```python
from build123d import *

# Parameters (mm, degrees)
F1_DEPTH = 10
F2_SIZE  = 5
F3_R     = 2.5
F4_DEPTH = 10
F5_R     = 1.5
F6_DEPTH = 12


with BuildPart() as f1:
    # F0 (on Front) → F1 (new body)
    with BuildSketch(Plane.XZ):
        with BuildLine():
            Line((-7, 0), (0, 0))
            Line((0, 0), (0, 30))
            Line((0, 30), (-20, 30))
            Line((-20, 30), (-20, 0))
            Line((-20, 0), (-13, 0))
            Line((-13, 0), (-13, 19.427699))
            ThreePointArc((-13, 19.427699), (-9.474739, 21.19446), (-7, 18.124513))
            Line((-7, 18.124513), (-7, 0))
        make_face()
    extrude(amount=F1_DEPTH)

    # F2
    f2_edges = [f1.edges().sort_by_distance(p)[0] for p in [
        (0, -5, 30),
        (-20, -5, 30),
    ]]
    chamfer(f2_edges, length=F2_SIZE)

    # F3 (on face) → F4 (cut)
    with BuildSketch(Plane.YZ):
        with Locations((-5, 16.878698)):
            Circle(F3_R)
        with Locations((-5, 7.148258)):
            Circle(F3_R)
    extrude(amount=-F4_DEPTH, mode=Mode.SUBTRACT)

    # F5 (on Front) → F6 (cut)
    with BuildSketch(Plane.XZ):
        with Locations((-16.984137, 21.757886)):
            Circle(F5_R)
        with Locations((-16.821511, 6.757886)):
            Circle(F5_R)
    extrude(amount=F6_DEPTH, mode=Mode.SUBTRACT)


solid = f1.part
```
Check sheet for the modelled part. Datum: model origin and axes. Units: mm. A direction names the side the tool comes from. Round coordinates to 2 decimals unless told otherwise and drop trailing zeros. Order: outer loops, then holes, each group sorted by start corner. A loop starts at its lowest first (then second) coordinate and runs counter-clockwise, first axis right, second up. Notation, with made-up numbers: (61, 58) - (101, 58) arc R24 cw to (101, 81) - close; hole circle Ø2 at (15, -31.75). An arc over 180 degrees is marked (long way). Write item = value, one per line.
Q1. Thickness scan on line 1 along Z through (x, y) = (-4.25, -5); line 2 along Z through (x, y) = (-4, -5); line 3 along X through (y, z) = (-4, 10.75). Record the ranges inside material, lowest first.
Computed:
line_1 = 0 to 4.65, 9.65 to 14.38, 19.38 to 29.25
line_2 = 0 to 4.65, 9.65 to 14.38, 19.38 to 29
line_3 = -20 to -13, -7 to 0
Q2. Section check C-C (x = -17.25). Record the boundary of the cut face in (y, z).
Computed:
outline = (-10, 0) - (0, 0) - (0, 5.32) - (-10, 5.32) - close; (-10, 8.2) - (0, 8.2) - (0, 20.28) - (-10, 20.28) - close; (-10, 23.23) - (0, 23.23) - (0, 27.75) - (-10, 27.75) - close
Q3. Section check B-B (y = -5). Record the boundary of the cut face in (x, z), and give its area (3 significant figures).
Computed:
outline = (-20, 0) - (-13, 0) - (-13, 19.43) arc R3.14 cw to (-7.26, 19.38) - (0, 19.38) - (0, 25) - (-5, 30) - (-15, 30) - (-20, 25) - close; (-7, 0) - (0, 0) - (0, 4.65) - (-7, 4.65) - close; (-7, 9.65) - (0, 9.65) - (0, 14.38) - (-7, 14.38) - close; hole circle Ø3 at (-16.98, 21.76); hole circle Ø3 at (-16.82, 6.76)
area = 367 mm^2
Q4. Draft check along Z on faces 4 (the face through (-18.483, -4.93, 21.824)), 5 (the face through (-6, 0, 15)), 6 (the face through (-3.451, -2.615, 7.899)), 7 (the face through (-4, -5, 0)). Enter one of: pulls with the +Z half, pulls with the -Z half, needs draft (parallel to the pull), parting line crosses it, or undercut.
Computed:
face_4 = undercut
face_5 = needs draft
face_6 = undercut
face_7 = pulls with the -Z half
Q5. Section check D-D (y = -1.75). Record the boundary of the cut face in (x, z), and give its area (3 significant figures).
Computed:
outline = (-20, 0) - (-13, 0) - (-13, 19.43) arc R3.14 cw to (-7, 18.12) - (-7, 0) - (0, 0) - (0, 25) - (-5, 30) - (-15, 30) - (-20, 25) - close; hole circle Ø3 at (-16.98, 21.76); hole circle Ø3 at (-16.82, 6.76)
area = 437 mm^2
Q6. Go/stop test with a flat-tipped pin: pin 1 (4.5 mm diameter, centred on y = -5, z = 16.88, fed in from +X). Record where the tip stops, or that it passes through.
Computed:
pin_1 = -13
Q7. Section check A-A (z = 13). Record the boundary of the cut face in (x, y).
Computed:
outline = (-20, -10) - (-13, -10) - (-13, 0) - (-20, 0) - close; (-7, -10) - (0, -10) - (0, 0) - (-7, 0) - close
Q8. Tool access check on faces 1 (the face through (-3.58, -3.66, 18.99)), 2 (the face through (0, -5, 12)), 3 (the face through (-7, -3, 9)). Record the directions out of +Z, -Z, +X, -X, +Y, -Y that give a thin tool (end or side, any length) a straight path to the whole face; none if there is none.
Computed:
face_1 = +X
face_2 = +Z, -Z, +X, +Y, -Y
face_3 = -Z, +Y, -Y
